```python
from build123d import *

# Parameters (mm, degrees)
SKETCH1_W                       = 38
SKETCH1_H                       = 50
BOSS_EXTRUDE1_DEPTH             = 25
BOSS_EXTRUDE8_DEPTH             = 10
FILLET1_R                       = 0.3
FILLET1_OF_MIRROR1_R            = 0.3
CUT_EXTRUDE7_REACH              = 77.873
SKETCH15_W                      = 45
SKETCH15_H                      = 29
BOSS_EXTRUDE2_DEPTH             = 38
SKETCH16_R                      = 11.1
CUT_EXTRUDE8_DEPTH              = 3.5
SKETCH17_R                      = 6.05
CUT_EXTRUDE9_DEPTH              = 19
SKETCH18_R                      = 7.5
SKETCH18_R_2                    = 6.05
CUT_EXTRUDE10_DEPTH             = 5.8
CUT_EXTRUDE11_START             = -15.8
CUT_EXTRUDE11_DEPTH             = 15.8
SKETCH20_R                      = 1.85
CUT_EXTRUDE12_DEPTH             = 19
CIRPATTERN1_COUNT               = 2
CIRPATTERN1_ANGLE               = 90
CIRPATTERN1_THE_OTHER_WAY_COUNT = 2
CIRPATTERN1_THE_OTHER_WAY_ANGLE = 90
SKETCH24_W                      = 15.3
SKETCH24_H                      = 21.6
SKETCH24_R                      = 1.85
CUT_EXTRUDE13_DEPTH             = 16
SKETCH25_R                      = 4.2
CUT_EXTRUDE14_DEPTH             = 101.421935127
SKETCH27_W                      = 22
SKETCH27_H                      = 43
CUT_EXTRUDE15_DEPTH             = 25


with BuildPart() as part:
    # Sketch1 → Boss-Extrude1 (new body)
    with BuildSketch(Plane.XY):
        with Locations((-19, 0)):
            Rectangle(SKETCH1_W, SKETCH1_H)
    boss_extrude1 = extrude(amount=BOSS_EXTRUDE1_DEPTH)

    # Sketch11 → Boss-Extrude8 (add)
    with BuildSketch(Plane(origin=(-28, 0, 0), x_dir=(0, 0, -1), z_dir=(1, 0, 0))):
        with BuildLine():
            Line((-5.0442209, -55.726230367), (-5.0442209, -29.776230367))
            ThreePointArc((-5.0442209, -29.776230367), (-4.915049594, -29.069123586), (-4.5442209, -28.453354711))
            ThreePointArc((-4.5442209, -28.453354711), (-4.310852684, -28.228443584), (-4.0442209, -28.044179559))
            ThreePointArc((-4.0442209, -28.044179559), (2.432940548, -29.34409424), (1.9670283, -35.933959519))
            Line((1.9670283, -35.933959519), (-4.9442209, -42.751230367))
            Line((-4.9442209, -42.751230367), (-2.13522154, -45.598952719))
            Line((-2.13522154, -45.598952719), (-1.423290952, -44.896702879))
            Line((-1.423290952, -44.896702879), (-2.827790632, -43.472841703))
            Line((-2.827790632, -43.472841703), (4.31462396, -36.427548823))
            ThreePointArc((4.31462396, -36.427548823), (4.819099677, -35.868688789), (5.255569039, -35.255243777))
            ThreePointArc((5.255569039, -35.255243777), (5.821779814, -34.120234879), (6.156782985, -32.896873642))
            ThreePointArc((6.156782985, -32.896873642), (6.148424754, -30.655377502), (5.379165125, -28.55))
            ThreePointArc((5.379165125, -28.55), (3.107671966, -26.234387817), (0, -25.304809472))
            ThreePointArc((0, -25.304809472), (-0.25, -25.3), (-0.5, -25.304809472))
            ThreePointArc((-0.5, -25.304809472), (-2.379635768, -25.65877443), (-4.074871702, -26.544492749))
            ThreePointArc((-4.074871702, -26.544492749), (-5.891365223, -28.673957334), (-6.5442209, -31.395730211))
            Line((-6.5442209, -31.395730211), (-6.5442209, -60.726230367))
            Line((-6.5442209, -60.726230367), (-4.6442209, -60.726230367))
            Line((-4.6442209, -60.726230367), (-4.6442209, -55.726230367))
            Line((-4.6442209, -55.726230367), (-5.0442209, -55.726230367))
        make_face()
        Polygon((-7.5442209, -60.726230367), (-6.5442209, -60.726230367), (-6.5442209, -31.395730211), (-6.5442209, -25), (-7.5442209, -25), (-7.5442209, -49.208689401), align=None)
        with BuildLine():
            ThreePointArc((5.255569039, -35.255243777), (4.819099677, -35.868688789), (4.31462396, -36.427548823))
            Line((4.31462396, -36.427548823), (10.04868827, -40.442583877))
            Line((10.04868827, -40.442583877), (10.04868827, -36.637851334))
            Line((10.04868827, -36.637851334), (5.379165125, -28.55))
            ThreePointArc((5.379165125, -28.55), (6.148424754, -30.655377502), (6.156782985, -32.896873642))
            Line((6.156782985, -32.896873642), (9.053935122, -37.914888341))
            Line((9.053935122, -37.914888341), (5.255569039, -35.255243777))
        make_face()
        with BuildLine():
            Line((-0.5, -25), (-0.5, -25.304809472))
            ThreePointArc((-0.5, -25.304809472), (-0.25, -25.3), (0, -25.304809472))
            Line((0, -25.304809472), (0, -25))
            Line((0, -25), (-0.5, -25))
        make_face()
        Polygon((-13.843719233, -25), (-7.5442209, -60.726230367), (-7.5442209, -49.208689401), (-11.812866009, -25), align=None)
    boss_extrude8 = extrude(amount=BOSS_EXTRUDE8_DEPTH)

    # Fillet1
    fillet1_edges = [part.edges().sort_by_distance(p)[0] for p in [
        (-23, -42.751230367, 4.9442209),
    ]]
    fillet(fillet1_edges, radius=FILLET1_R)

    # Mirror1: Boss-Extrude1, Boss-Extrude8 across plane
    add(boss_extrude1.mirror(Plane(origin=(0, 0, 0), x_dir=(0, 0, 1), z_dir=(1, 0, 0))))
    add(boss_extrude8.mirror(Plane(origin=(0, 0, 0), x_dir=(0, 0, 1), z_dir=(1, 0, 0))))

    # Fillet1 of Mirror1
    fillet1_of_mirror1_edges = [part.edges().sort_by_distance(p)[0] for p in [
        (23, -42.751230367, 4.9442209),
    ]]
    fillet(fillet1_of_mirror1_edges, radius=FILLET1_OF_MIRROR1_R)

    # Sketch15 → Cut-Extrude7 (cut, up to next)
    with BuildSketch(Plane(origin=(0, 0, 0), x_dir=(-1, 0, 0), z_dir=(0, 0, -1)), mode=Mode.PRIVATE) as cut_extrude7_sk1:
        with Locations((15.5, 0)):
            Rectangle(SKETCH15_W, SKETCH15_H)
    cut_extrude7_tool1 = extrude(cut_extrude7_sk1.sketch, amount=-CUT_EXTRUDE7_REACH, mode=Mode.PRIVATE) & part.part
    add(cut_extrude7_tool1.solids().sort_by_distance((-15.5, 0, 0))[0], mode=Mode.SUBTRACT)

    # Sketch2 → Boss-Extrude2 (add)
    with BuildSketch(Plane.ZY.offset(-28)):
        Polygon((32, 7.541451884), (25, 3.5), (25, -3.5), (32, -7.541451884), align=None)
    extrude(amount=BOSS_EXTRUDE2_DEPTH)

    # Sketch16 → Cut-Extrude8 (cut)
    with BuildSketch(Plane.ZY.offset(-7)):
        with Locations((12.5, 0)):
            Circle(SKETCH16_R)
    extrude(amount=-CUT_EXTRUDE8_DEPTH, mode=Mode.SUBTRACT)

    # Sketch17 → Cut-Extrude9 (cut)
    with BuildSketch(Plane.ZY.offset(-10.5)):
        with Locations((12.5, 0)):
            Circle(SKETCH17_R)
    extrude(amount=-CUT_EXTRUDE9_DEPTH, mode=Mode.SUBTRACT)

    # Sketch18 → Cut-Extrude10 (cut)
    # profile 1 of 3: a face of its own
    with BuildSketch(Plane.ZY.offset(-29.5)):
        with BuildLine():
            ThreePointArc((12.5, -7.5), (5, 0), (12.5, 7.5))
            Line((12.5, 7.5), (0, 7.5))
            Line((0, 7.5), (0, -7.5))
            Line((0, -7.5), (12.5, -7.5))
        make_face()
    # profile 2 of 3: a face of its own
    with BuildSketch(Plane.ZY.offset(-29.5)):
        with Locations((12.5, 0)):
            Circle(SKETCH18_R)
        with Locations((12.5, 0)):
            Circle(SKETCH18_R_2, mode=Mode.SUBTRACT)
    # profile 3 of 3: a face of its own
    with BuildSketch(Plane.ZY.offset(-29.5)):
        with Locations((12.5, 0)):
            Circle(SKETCH18_R_2)
    extrude(amount=-CUT_EXTRUDE10_DEPTH, mode=Mode.SUBTRACT)

    # Sketch19 → Cut-Extrude11 (cut)
    with BuildSketch(Plane(origin=(29.5, 0, 0), x_dir=(0, 0, -1), z_dir=(1, 0, 0)).offset(CUT_EXTRUDE11_START)):
        with BuildLine():
            Line((-12.5, 6.05), (0, 6.05))
            Line((0, 6.05), (0, -6.05))
            Line((0, -6.05), (-12.5, -6.05))
            ThreePointArc((-12.5, -6.05), (-18.55, 0), (-12.5, 6.05))
        make_face()
    extrude(amount=CUT_EXTRUDE11_DEPTH, mode=Mode.SUBTRACT)

    # Sketch20 → Cut-Extrude12 (cut)
    with BuildSketch(Plane.ZY.offset(-10.5)):
        with Locations((4.5, 0)):
            Circle(SKETCH20_R)
    cut_extrude12 = extrude(amount=-CUT_EXTRUDE12_DEPTH, mode=Mode.SUBTRACT)

    # CirPattern1: Cut-Extrude12 ×2 about axis
    cirpattern1_axis = Axis((29.5, 0, 12.5), (-1, 0, 0))
    for i in range(1, CIRPATTERN1_COUNT):
        add(cut_extrude12.rotate(cirpattern1_axis, i * CIRPATTERN1_ANGLE / (CIRPATTERN1_COUNT - 1)), mode=Mode.SUBTRACT)

    # CirPattern1 the other way: Cut-Extrude12 ×2 about axis
    cirpattern1_the_other_way_axis = Axis((29.5, 0, 12.5), (1, 0, 0))
    for i in range(1, CIRPATTERN1_THE_OTHER_WAY_COUNT):
        add(cut_extrude12.rotate(cirpattern1_the_other_way_axis, i * CIRPATTERN1_THE_OTHER_WAY_ANGLE / (CIRPATTERN1_THE_OTHER_WAY_COUNT - 1)), mode=Mode.SUBTRACT)

    # Sketch24 → Cut-Extrude13 (cut)
    with BuildSketch(Plane(origin=(13.7, 0, 0), x_dir=(0, 0, -1), z_dir=(1, 0, 0))):
        with Locations((-7.65, 0)):
            Rectangle(SKETCH24_W, SKETCH24_H)
        with Locations(Location((-12.5, -8, 0), (0, 0, 90))):
            Circle(SKETCH24_R, mode=Mode.SUBTRACT)
        with Locations(Location((-12.5, 8, 0), (0, 0, 270))):
            Circle(SKETCH24_R, mode=Mode.SUBTRACT)
    extrude(amount=CUT_EXTRUDE13_DEPTH, mode=Mode.SUBTRACT)

    # Sketch25 → Cut-Extrude14 (cut, through all)
    with BuildSketch(Plane.ZY.offset(-35.3)):
        with Locations((12.5, 0)):
            Circle(SKETCH25_R)
    extrude(amount=-CUT_EXTRUDE14_DEPTH, mode=Mode.SUBTRACT)

    # Sketch27 → Cut-Extrude15 (cut)
    with BuildSketch(Plane(origin=(0, 0, 0), x_dir=(-1, 0, 0), z_dir=(0, 0, -1))):
        with Locations((27, 0)):
            Rectangle(SKETCH27_W, SKETCH27_H)
    extrude(amount=-CUT_EXTRUDE15_DEPTH, mode=Mode.SUBTRACT)


solid = part.part
```
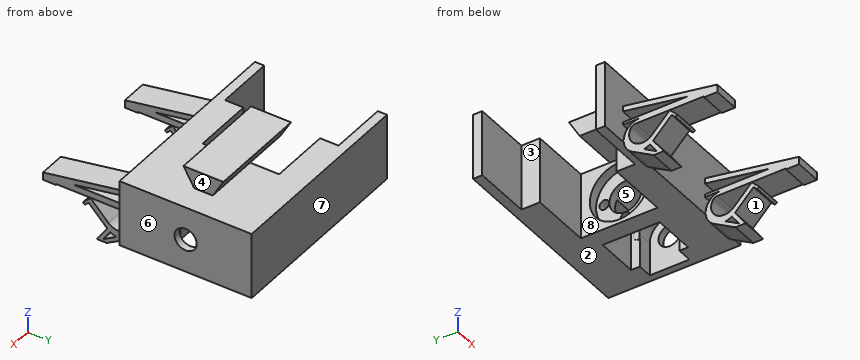
Check sheet for the modelled part. Datum: model origin and axes. Units: mm. Face numbers are marked on the shaded views. A direction names the side the tool comes from. Give positions to 0.01 mm unless a question says otherwise; leave off trailing zeros. Loops run counter-clockwise (first coordinate to the right, second up) from the corner with the lowest first, then second, coordinate; pieces in that order, holes last. Notation, with made-up numbers: M 55.5,-18 L 105.5,-18 A26 ccw 105.5,-2 Z; hole C -10,-24.5 d6. An arc over 180 degrees is marked long. Answer in a Markdown table with one row per item.
1) Mould release check, pull along Y, two halves, no side actions. Record for the marked faces 6, 7 and 8: released by +Y, released by -Y, zero draft, split by the parting line, or undercut.
Solutions:
| item | result |
|---|---|
| face 6 | zero draft |
| face 7 | released by +Y |
| face 8 | undercut |
2) Depth check by flat-ended pin: pin 1 (12 mm diameter, centred on y = -40, z = 7, fed in from +X); pin 2 (3 mm diameter, centred on y = 9, z = 12, fed in from -X); pin 3 (6 mm diameter, centred on x = 18.5, y = -7, fed in from -Z). Enter the tip coordinate at first touch or a pass-through.
Solutions:
| item | result |
|---|---|
| pin 1 | stops at x = 28 |
| pin 2 | stops at x = 10.5 |
| pin 3 | stops at z = 15.3 |
3) Cross-section at D-D (y = -18.5). Enter the section's corners in (x, z), plus the area to 3 significant figures.
Solutions:
| item | result |
|---|---|
| outline | M -16,0 L 38,0 L 38,25 L -16,25 Z |
| area | 1,350 mm^2 |
4) Cross-section at A-A (y = 0). Enter the section's corners in (x, z).
Solutions:
| item | result |
|---|---|
| outline | M -10,25 L 7,25 L 7,23.6 L 10.5,23.6 L 10.5,18.55 L 29.5,18.55 L 29.5,20 L 35.3,20 L 35.3,16.7 L 38,16.7 L 38,25 L 28,25 L 28,32 L -10,32 Z; M 7,0 L 13.7,0 L 13.7,2.65 L 10.5,2.65 L 10.5,1.4 L 7,1.4 Z; M 10.5,6.35 L 13.7,6.35 L 13.7,6.45 L 10.5,6.45 Z; M 35.3,0 L 38,0 L 38,8.3 L 35.3,8.3 Z |
5) Cross-section at C-C (x = -1.5). Enter the section's corners in (y, z), plus the area to 3 significant figures.
Solutions:
| item | result |
|---|---|
| outline | M -25,0 L -14.5,0 L -14.5,25 L -25,25 Z; M -7.54,32 L -3.5,25 L 3.5,25 L 7.54,32 Z; M 14.5,0 L 25,0 L 25,25 L 14.5,25 Z |
| area | 602 mm^2 |
6) Thickness scan on line 1 (Z direction, x = 12.4, y = 8); line 2 (X direction, y = 4, z = 6); line 3 (Y direction, x = 12.15, z = 4.5). Record the ranges inside material, lowest first.
Solutions:
| item | result |
|---|---|
| line 1 | z = 0 to 10.65, 14.35 to 25 |
| line 2 | x = 10.5 to 13.7, 35.3 to 38 |
| line 3 | y = -25 to -1.85, 1.85 to 25 |
7) Cross-section at B-B (x = -19.5). Count the separate pieces of the cut face and the enclosed holes in it, plus the area to 3 significant figures.
Solutions:
| item | result |
|---|---|
| separate pieces | 2 |
| enclosed holes | 3 |
| area | 408 mm^2 |
8) Tool access check on the marked faces 1, 2, 3, 4 and 5. Record the directions out of +Z, -Z, +X, -X, +Y, -Y that give a thin tool (end or side, any length) a straight path to the whole face; none if there is none.
Solutions:
| item | result |
|---|---|
| face 1 | +X, -X |
| face 2 | -Z, +X, -X, +Y |
| face 3 | +Z, -Z, -X |
| face 4 | +Z, +X, +Y, -Y |
| face 5 | -X |
